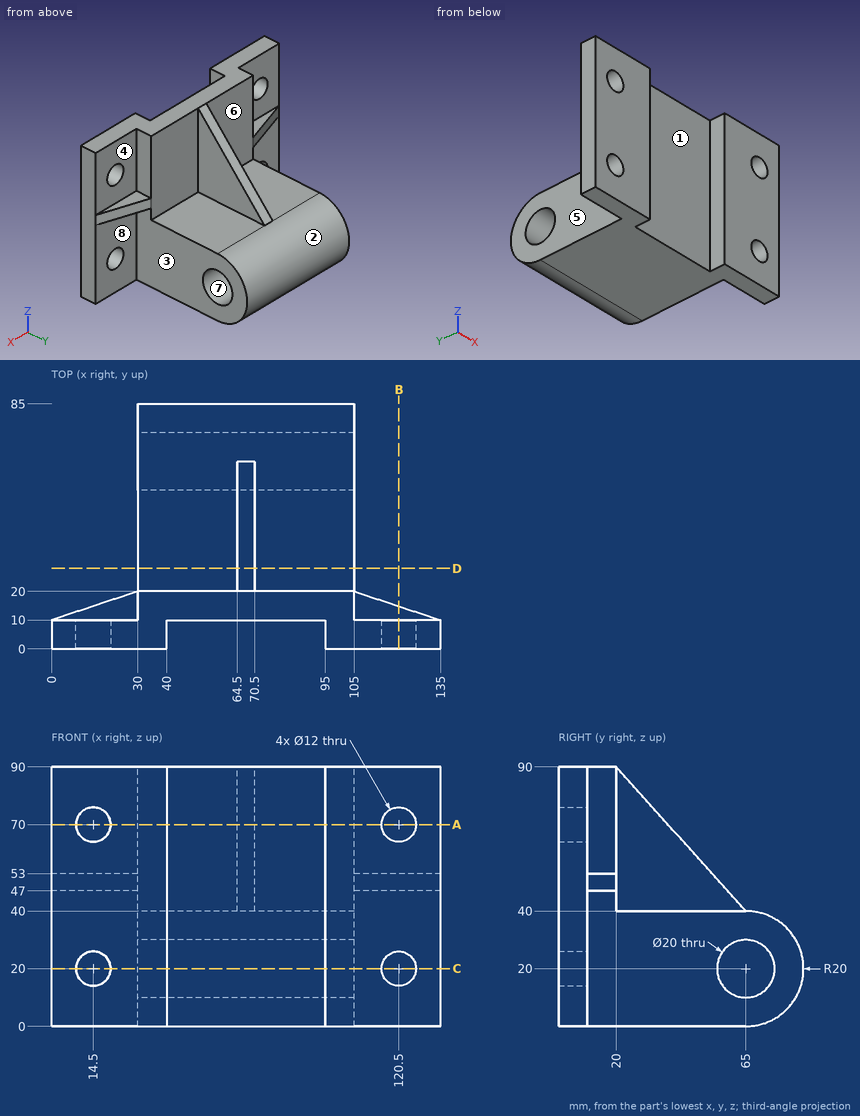
Source: three-view drawing plus pictorial views. Frame: mm from the lowest corner of the part. A direction names the side the tool comes from. Give positions to 0.01 mm unless a question says otherwise; leave off trailing zeros. Write each loop counter-clockwise with the first axis right and the second up, starting at its lowest first coordinate (ties: lowest second). Pieces come first, ordered by that corner, then holes.
(1) Cut plane D-D, the plane y = 28. Return loops of the section in (x, z).
(2) Cut plane A-A, the plane z = 70. Return loops of the section in (x, y), then the cut area to 3 significant figures.
(3) First-contact query: P1, Ø23.5, axis at y = 64, z = 27, coming from the -X side; P2, Ø24, axis at x = 114.5, z = 14, coming from the +Y side; P3, Ø5, axis at x = 70.5, z = 59.5, coming from the +Y side. Flat tips, straight axial feed; report the tip coordinate or a pass-through.
(4) Ray query, line 1 (Z direction, x = 120.5, y = 6); line 2 (Z direction, x = 70, y = 65.5); line 3 (Z direction, x = 50, y = 29). Return the intervals inside material, ascending.
(5) Cut plane C-C, the plane z = 20. Return loops of the section in (x, y), then the cut area to 4 significant figures.
(6) Cut plane B-B, the plane x = 120.5. Return loops of the section in (y, z), then the cut area to 3 significant figures.
(7) Mould query, pull axis X, two halves, no side actions, for the marked faces 1, 2 and 3. Classes: released by +X, released by -X, zero draft, split by the parting line, or undercut.
(8) Access query for the marked faces 4, 5, 6, 7 and 8. Directions: +Z, -Z, +X, -X, +Y, -Y. A direction counts if a zero-diameter tool reaches every point of the face in a straight line with its end or side. Return the directions, or none.
Values follow:
1. outline: (30, 0) - (105, 0) - (105, 40) - (70.5, 40) - (70.5, 81.11) - (64.5, 81.11) - (64.5, 40) - (30, 40) - close
2. outline: (0, 0) - (8.5, 0) - (8.5, 10) - (0, 10) - close; (20.5, 0) - (40, 0) - (40, 10) - (95, 10) - (95, 0) - (114.5, 0) - (114.5, 10) - (105, 10) - (105, 20) - (70.5, 20) - (70.5, 38) - (64.5, 38) - (64.5, 20) - (30, 20) - (30, 10) - (20.5, 10) - close; (126.5, 0) - (135, 0) - (135, 10) - (126.5, 10) - close
2. area: 1,420 mm2
3. P1: stops at x = 30
3. P2: stops at y = 85
3. P3: stops at y = 49.7
4. line 1: z = 0 to 14, 26 to 64, 76 to 90
4. line 2: z = 0.01 to 10.01, 29.99 to 39.99
4. line 3: z = 0 to 40
5. outline: (0, 0) - (8.5, 0) - (8.5, 10) - (0, 10) - close; (20.5, 0) - (40, 0) - (40, 10) - (95, 10) - (95, 0) - (114.5, 0) - (114.5, 10) - (105, 10) - (105, 55) - (30, 55) - (30, 10) - (20.5, 10) - close; (30, 75) - (105, 75) - (105, 85) - (30, 85) - close; (126.5, 0) - (135, 0) - (135, 10) - (126.5, 10) - close
5. area: 4,685 mm2
6. outline: (0, 0) - (10, 0) - (10, 14) - (0, 14) - close; (0, 26) - (10, 26) - (10, 47) - (14.83, 47) - (14.83, 53) - (10, 53) - (10, 64) - (0, 64) - close; (0, 76) - (10, 76) - (10, 90) - (0, 90) - close
6. area: 689 mm2
7. face 1: undercut
7. face 2: zero draft
7. face 3: released by +X
8. face 4: +Z, +X, +Y
8. face 5: -Z, -X, +Y
8. face 6: +Z, -X, +Y
8. face 7: +X, -X
8. face 8: -Z, +X, +Y
